```python
from build123d import *

# Parameters (mm, degrees)
F1_DEPTH = 3


with BuildPart() as f1:
    # F0 (on Front) → F1 (new body)
    with BuildSketch(Plane.XZ):
        Polygon((93.15, -13.522226), (106.45, -13.522226), (106.45, -10.522226), (116.75, -10.522226), (116.75, -3.352226), (119.75, -3.352226), (119.75, 6.813774), (116.75, 6.813774), (116.75, 16.979774), (119.75, 16.979774), (119.75, 27.145774), (116.75, 27.145774), (116.75, 37.311774), (119.75, 37.311774), (119.75, 47.477774), (-119.75, 47.477774), (-119.75, 37.311774), (-116.75, 37.311774), (-116.75, 27.145774), (-119.75, 27.145774), (-119.75, 16.979774), (-116.75, 16.979774), (-116.75, 6.813774), (-119.75, 6.813774), (-119.75, -3.352226), (-116.75, -3.352226), (-116.75, -13.522226), (-106.45, -13.522226), (-106.45, -10.522226), (-93.15, -10.522226), (-93.15, -13.522226), (-79.85, -13.522226), (-79.85, -10.522226), (-66.55, -10.522226), (-66.55, -13.522226), (-53.25, -13.522226), (-53.25, -10.522226), (-39.95, -10.522226), (-39.95, -13.522226), (-26.65, -13.522226), (-26.65, -10.522226), (-13.35, -10.522226), (-13.35, -13.522226), (-0.05, -13.522226), (-0.05, -10.522226), (0.05, -10.522226), (13.35, -10.522226), (13.35, -13.522226), (26.65, -13.522226), (26.65, -10.522226), (39.95, -10.522226), (39.95, -13.522226), (53.25, -13.522226), (53.25, -10.522226), (66.55, -10.522226), (66.55, -13.522226), (79.85, -13.522226), (79.85, -10.522226), (93.15, -10.522226), align=None)
    extrude(amount=F1_DEPTH)


solid = f1.part
```
Work out the finished part from the listing and answer in its coordinate system (mm). Coordinates: 2 decimals unless noted, no trailing zeros. Loops run counter-clockwise (first coordinate to the right, second up) from the corner with the lowest first, then second, coordinate; pieces in that order, holes last. Notation, with made-up numbers: (83, -28.5) - (99, -28.5) arc R12 ccw to (99, -13.5) - close; hole circle Ø11 at (40.25, -1). An arc over 180 degrees is marked (long way). Use a Markdown table: item, result.
Item 1: Find section B-B, the plane x = -45. Determine the outline of the cut face in (y, z), and give its area (3 significant figures).
Evaluation:
| item | result |
|---|---|
| outline | (-3, -10.52) - (0, -10.52) - (0, 47.48) - (-3, 47.48) - close |
| area | 174 mm2 |
Item 2: Consider probe 1 along X at (y, z) = (-1.1, 7.5); probe 2 along Z at (x, y) = (86.5, -2.5). Determine where each line is inside the solid, lowest interval first. Write a range as from..to.
Evaluation:
| item | result |
|---|---|
| probe 1 | x = -116.75..116.75 |
| probe 2 | z = -10.52..47.48 |
Item 3: Given pin 1 Ø10 at (x, z) = (30, 15.5) entering from +Y; pin 2 Ø1.5 at (y, z) = (-1.5, -11.5) entering from +X; pin 3 Ø1.5 at (x, y) = (-98, -1) entering from -Z; pin 4 Ø1.5 at (y, z) = (-2, -12.5) entering from -X, each flat-ended and moving along its own axis, determine where each tip first touches the part or whether it passes through.
Evaluation:
| item | result |
|---|---|
| pin 1 | stops at y = 0 |
| pin 2 | stops at x = 106.45 |
| pin 3 | stops at z = -10.52 |
| pin 4 | stops at x = -116.75 |
Item 4: Find section A-A, the plane z = -6. Determine the outline of the cut face in (x, y), and give its area (4 significant figures).
Evaluation:
| item | result |
|---|---|
| outline | (-116.75, -3) - (116.75, -3) - (116.75, 0) - (-116.75, 0) - close |
| area | 700.5 mm2 |
